Input: part model. Units: mm. Frame: model coordinates. Face numbers are marked on the shaded views. A direction names the side the tool comes from. Give positions to 0.01 mm unless a question says otherwise; leave off trailing zeros. Order: outer loops, then holes, each group sorted by start corner. A loop starts at its lowest first (then second) coordinate and runs counter-clockwise, first axis right, second up. Notation, with made-up numbers: (-10.5, 71.5) - (-6.5, 71.5) arc R20 ccw to (-6.5, 103.5) - close; hole circle Ø6 at (58, 51). An arc over 180 degrees is marked (long way). Use a Markdown table: item, result.
from build123d import *

# Parameters (mm, degrees)
SKETCH001_R        = 1.7
POCKET_DEPTH       = 157.778767
SKETCH002_R        = 2.95
POCKET001_DEPTH    = 6
SKETCH003_R        = 1.7
POCKET002_DEPTH    = 169.059555
SKETCH004_R        = 2.95
POCKET003_DEPTH    = 4
POLARPATTERN_COUNT = 3


with BuildPart() as part:
    # Sketch → Revolution (revolve)
    with BuildSketch(Plane.XZ):
        with BuildLine():
            Line((15, 9.990992), (15, 3.15))
            Line((15, 3.15), (0, 3.15))
            Line((0, 3.15), (0, 0))
            Line((0, 0), (25, 0))
            Line((25, 0), (25, 13.719212))
            ThreePointArc((15, 9.990992), (20.086685, 11.622592), (25, 13.719212))
        make_face()
    revolve(axis=Axis((0, 0, 0), (0, 0, 1)))

    # Sketch001 (on Face3 of Revolution) → Pocket (cut, through all)
    with BuildSketch(Plane(origin=(0, 0, 0), x_dir=(1, 0, 0), z_dir=(0, 0, -1))):
        with Locations((0, -20)):
            Circle(SKETCH001_R)
    pocket = extrude(amount=-POCKET_DEPTH, mode=Mode.SUBTRACT)

    # Sketch002 (on DatumPlane) → Pocket001 (cut)
    with BuildSketch(Plane.XY.offset(14)):
        with Locations((0, 20)):
            Circle(SKETCH002_R)
    pocket001 = extrude(amount=-POCKET001_DEPTH, mode=Mode.SUBTRACT)

    # Sketch003 → Pocket002 (cut, through all)
    with BuildSketch(Plane.XZ):
        with Locations((0, 7.65)):
            Circle(SKETCH003_R)
    pocket002 = extrude(amount=POCKET002_DEPTH, mode=Mode.SUBTRACT)

    # Sketch004 (on DatumPlane) → Pocket003 (cut)
    with BuildSketch(Plane.XZ.offset(25)):
        with Locations((0, 7.65)):
            Circle(SKETCH004_R)
    pocket003 = extrude(amount=-POCKET003_DEPTH, mode=Mode.SUBTRACT)

    # PolarPattern: Pocket, Pocket001, Pocket002, Pocket003 ×3 about axis
    polarpattern_axis = Axis((0, 0, 0), (0, 0, -1))
    for i in range(1, POLARPATTERN_COUNT):
        add(pocket.rotate(polarpattern_axis, i * 360 / POLARPATTERN_COUNT), mode=Mode.SUBTRACT)
        add(pocket001.rotate(polarpattern_axis, i * 360 / POLARPATTERN_COUNT), mode=Mode.SUBTRACT)
        add(pocket002.rotate(polarpattern_axis, i * 360 / POLARPATTERN_COUNT), mode=Mode.SUBTRACT)
        add(pocket003.rotate(polarpattern_axis, i * 360 / POLARPATTERN_COUNT), mode=Mode.SUBTRACT)


solid = part.part
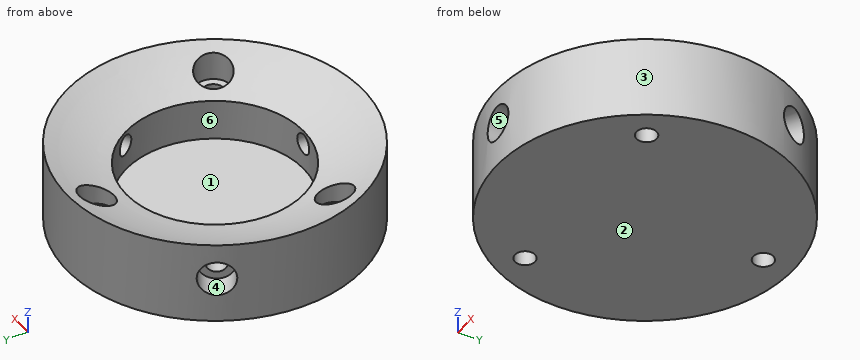
1. Section query B-B (z = 2). Return loops of the section in (x, y), then the cut area to 3 significant figures.
Response:
| item | result |
|---|---|
| outline | circle Ø50 at (0, 0); hole circle Ø3.4 at (-17.32, -10); hole circle Ø3.4 at (0, 20); hole circle Ø3.4 at (17.32, -10) |
| area | 1,940 mm^2 |
2. Section query A-A (x = -17.5). State how many separate pieces and enclosed holes the cut face has, then the cut area to 3 significant figures.
Response:
| item | result |
|---|---|
| separate pieces | 2 |
| enclosed holes | 1 |
| area | 353 mm^2 |
3. Material intervals for line 1 along Y through (x, z) = (0, 5.5); line 2 along X through (y, z) = (20, 4.5); line 3 along X through (y, z) = (-10, 9.9), sorted ascending.
Response:
| item | result |
|---|---|
| line 1 | y = -21 to -15, 15 to 18.3, 21.7 to 25 |
| line 2 | x = -15 to -1.7, 1.7 to 15 |
| line 3 | x = -22.91 to -20.27, -14.37 to -11.18, 11.18 to 14.37, 20.27 to 22.91 |
4. Set-up query: the marked faces 4, 5 and 6. Return all of +Z, -Z, +X, -X, +Y, -Y with unobstructed straight access to the full face (end or side cutting, diameter ignored); none if empty.
Response:
| item | result |
|---|---|
| face 4 | none |
| face 5 | -Y |
| face 6 | +Z |
5. Mould query, pull axis Y, two halves, no side actions, for the marked faces 1, 2 and 3. Classes: pulls with the +Y half, pulls with the -Y half, needs draft (parallel to the pull), parting line crosses it, or undercut.
Response:
| item | result |
|---|---|
| face 1 | undercut |
| face 2 | needs draft |
| face 3 | parting line crosses it |
6. Pin query (flat end, axial travel): pin 1 (8 mm diameter, centred on y = -10, z = 2.5, fed in from +X); pin 2 (2 mm diameter, centred on x = -17.32, y = -10, fed in from +Z); pin 3 (2 mm diameter, centred on x = 0, z = 7.65, fed in from +Y); pin 4 (8 mm diameter, centred on y = -9.5, z = 10, fed in from -X). Return the tip coordinate at first contact, or that it passes through.
Response:
| item | result |
|---|---|
| pin 1 | stops at x = 24.27 |
| pin 2 | passes through |
| pin 3 | stops at y = 25 |
| pin 4 | stops at x = -24.39 |
